For this review, take the finished solid that the model builds, in its own axes (mm). A direction names the side the tool comes from. Give positions to 0.01 mm unless a question says otherwise; leave off trailing zeros. Loops run counter-clockwise (first coordinate to the right, second up) from the corner with the lowest first, then second, coordinate; pieces in that order, holes last.
```python
from build123d import *

# Parameters (mm, degrees)
F0_W     = 42.3
F0_H     = 42.3
F0_R     = 1.5
F0_R_2   = 11
F0_R_3   = 2.5
F1_DEPTH = 34
F2_DEPTH = 2
F3_DEPTH = 20
F4_SIZE  = 5.5
F5_SIZE  = 0.2
F6_W     = 16
F6_H     = 12
F7_DEPTH = 6.5


with BuildPart() as f1:
    # F0 (on Top) → F1 (new body)
    with BuildSketch(Plane.XY):
        Rectangle(F0_W, F0_H)
        with Locations((-15.5, -15.5)):
            Circle(F0_R, mode=Mode.SUBTRACT)
        with Locations((15.5, -15.5)):
            Circle(F0_R, mode=Mode.SUBTRACT)
        with Locations((-15.5, 15.5)):
            Circle(F0_R, mode=Mode.SUBTRACT)
        Circle(F0_R_2, mode=Mode.SUBTRACT)
        with Locations((15.5, 15.5)):
            Circle(F0_R, mode=Mode.SUBTRACT)
        Circle(F0_R_2)
        Circle(F0_R_3, mode=Mode.SUBTRACT)
        Circle(F0_R_3)
    extrude(amount=F1_DEPTH)

    # F0 (on Top) → F2 (join)
    with BuildSketch(Plane.XY):
        Circle(F0_R_2)
        Circle(F0_R_3, mode=Mode.SUBTRACT)
    extrude(amount=-F2_DEPTH)

    # F0 (on Top) → F3 (join)
    with BuildSketch(Plane.XY):
        Circle(F0_R_3)
    extrude(amount=-F3_DEPTH)

    # F4
    f4_edges = [f1.edges().sort_by_distance(p)[0] for p in [
        (-21.15, -21.15, 17),
        (21.15, -21.15, 17),
        (21.15, 21.15, 17),
        (-21.15, 21.15, 17),
    ]]
    chamfer(f4_edges, length=F4_SIZE)

    # F5
    f5_edges = [f1.edges().sort_by_distance(p)[0] for p in [
        (-2.5, 0, -20),
    ]]
    chamfer(f5_edges, length=F5_SIZE)

    # F6 (on face) → F7 (join)
    with BuildSketch(Plane.YZ.offset(21.15)):
        with Locations((0, 28)):
            Rectangle(F6_W, F6_H)
    extrude(amount=F7_DEPTH)


solid = f1.part
```
Item 1: The part is to be moulded in two halves that separate along X. For faces 4 (the flat face through (27.65, 0, 28)), 5 (the cylindrical face through (-0.54, -2.44, -10.78)), 6 (the flat face through (0, 0, -20)), 7 (the cylindrical face through (14, -15.43, 16.76)), say which applies: released by +X, released by -X, zero draft, split by the parting line, or undercut.
Answer:
face 4: released by +X
face 5: split by the parting line
face 6: zero draft
face 7: undercut
Item 2: Take a section at C-C on x = 0. Give the boundary of the cut face in (y, z).
Answer:
outline: (-21.15, 0) - (-11, 0) - (-11, -2) - (-2.5, -2) - (-2.5, -19.8) - (-2.3, -20) - (2.3, -20) - (2.5, -19.8) - (2.5, -2) - (11, -2) - (11, 0) - (21.15, 0) - (21.15, 34) - (-21.15, 34) - close
Item 3: Take a section at B-B on y = 0. Give the boundary of the cut face in (x, z), and give its area (3 significant figures).
Answer:
outline: (-21.15, 0) - (-11, 0) - (-11, -2) - (-2.5, -2) - (-2.5, -19.8) - (-2.3, -20) - (2.3, -20) - (2.5, -19.8) - (2.5, -2) - (11, -2) - (11, 0) - (21.15, 0) - (21.15, 22) - (27.65, 22) - (27.65, 34) - (-21.15, 34) - close
area: 1,650 mm2
Item 4: For L1, parallel to Y at x = 15.5, z = 14; L2, parallel to X at y = 16, z = 16; L3, parallel to X at y = -15, z = 24, list the stretches that pass through material, from the lowest coordinate up.
Answer:
L1: y = -21.15 to -17, -14 to 14, 17 to 21.15
L2: x = -20.8 to -16.91, -14.09 to 14.09, 16.91 to 20.8
L3: x = -21.15 to -16.91, -14.09 to 14.09, 16.91 to 21.15
Item 5: Take a section at D-D on x = 6. Give the boundary of the cut face in (y, z), and give its area (3 significant figures).
Answer:
outline: (-21.15, 0) - (-9.22, 0) - (-9.22, -2) - (9.22, -2) - (9.22, 0) - (21.15, 0) - (21.15, 34) - (-21.15, 34) - close
area: 1,480 mm2
Item 6: Clearance check with flat-ended pins moving along their axes: pin 1 Ø2.5 at (x, y) = (-15.5, 15.5) entering from -Z; pin 2 Ø2 at (x, z) = (23.5, 25) entering from -Y; pin 3 Ø17.5 at (x, y) = (1.5, 3) entering from -Z; pin 4 Ø5 at (x, y) = (-15.5, -15.5) entering from -Z. State where each tip first meets the part, or that it passes through.
Answer:
pin 1: passes through
pin 2: stops at y = -8
pin 3: stops at z = -20
pin 4: stops at z = 0
Item 7: Tool access review of faces 1 (the cylindrical face through (-2.38, -10.74, -0.99)), 2 (the flat face through (24, -8, 28)), 3 (the flat face through (24, 0, 22)): name each direction out of +Z, -Z, +X, -X, +Y, -Y from which nothing blocks a thin tool from reaching the whole face with its end or side.
Answer:
face 1: -Z
face 2: +Z, -Z, +X, -Y
face 3: -Z, +X, +Y, -Y
Item 8: Take a section at A-A on z = 29.5. Give the boundary of the cut face in (x, y), and give its area (3 significant figures).
Answer:
outline: (-21.15, -15.65) - (-15.65, -21.15) - (15.65, -21.15) - (21.15, -15.65) - (21.15, -8) - (27.65, -8) - (27.65, 8) - (21.15, 8) - (21.15, 15.65) - (15.65, 21.15) - (-15.65, 21.15) - (-21.15, 15.65) - close; hole circle Ø3 at (-15.5, -15.5); hole circle Ø3 at (-15.5, 15.5); hole circle Ø3 at (15.5, -15.5); hole circle Ø3 at (15.5, 15.5)
area: 1,800 mm2
